Design review of the part built by this model. Coordinates are the model's own, in mm. Face numbers are marked on the shaded views. A direction names the side the tool comes from. Coordinates: 2 decimals unless noted, no trailing zeros. Write each loop counter-clockwise with the first axis right and the second up, starting at its lowest first coordinate (ties: lowest second). Pieces come first, ordered by that corner, then holes. Notation, with made-up numbers: (62, 26) - (75, 26) arc R28 cw to (75, 62) - close; hole circle Ø10 at (22, 3.5). An arc over 180 degrees is marked (long way). Answer as a JSON object with one key per item and string values.
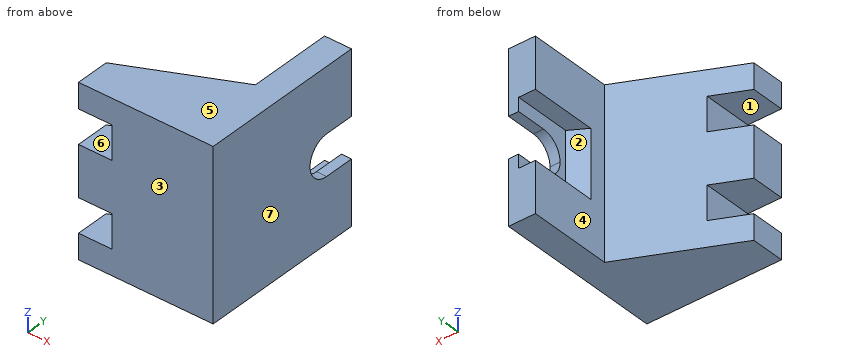
```python
from build123d import *

# Parameters (mm, degrees)
EXTRUDE_1_DEPTH          = 50
SKETCH_2_W               = 10
SKETCH_2_H               = 10
CUT_EXTRUDE_1_DEPTH      = 74.484692283
CUT_EXTRUDE_2_DEPTH      = 50
CUT_EXTRUDE_3_DEPTH      = 10
CUT_EXTRUDE_3_DEPTH_BACK = 10


with BuildPart() as part:
    # Эскиз1 → Бобышка-Вытянуть1 (new body)
    with BuildSketch(Plane.XY):
        Polygon((20, 25), (12, 25), (12, 0), (-20, -15), (-20, -25), (20, -25), align=None)
    extrude(amount=EXTRUDE_1_DEPTH)

    # Эскиз2 → Вырез-Вытянуть1 (cut, through all)
    with BuildSketch(Plane.XZ.offset(25)):
        with Locations((-15, 12.5)):
            Rectangle(SKETCH_2_W, SKETCH_2_H)
        with Locations((-15, 37.5)):
            Rectangle(SKETCH_2_W, SKETCH_2_H)
    extrude(amount=-CUT_EXTRUDE_1_DEPTH, mode=Mode.SUBTRACT)

    # Эскиз3 → Вырез-Вытянуть2 (cut)
    with BuildSketch(Plane(origin=(20, 0, 0), x_dir=(0, 0, -1), z_dir=(1, 0, 0))):
        with BuildLine():
            Line((-19, 25), (-25, 25))
            Line((-25, 25), (-25, 22))
            ThreePointArc((-25, 22), (-20.757359313, 20.242640687), (-19, 16))
            Line((-19, 16), (-19, 25))
        make_face()
        with BuildLine():
            ThreePointArc((-19, 16), (-20.757359313, 20.242640687), (-25, 22))
            Line((-25, 22), (-25, 10))
            ThreePointArc((-25, 10), (-20.757359313, 11.757359313), (-19, 16))
        make_face()
        with BuildLine():
            Line((-25, 10), (-25, 22))
            ThreePointArc((-25, 22), (-29.242640687, 20.242640687), (-31, 16))
            ThreePointArc((-31, 16), (-29.242640687, 11.757359313), (-25, 10))
        make_face()
        with BuildLine():
            Line((-25, 22), (-25, 25))
            Line((-25, 25), (-31, 25))
            Line((-31, 25), (-31, 16))
            ThreePointArc((-31, 16), (-29.242640687, 20.242640687), (-25, 22))
        make_face()
    extrude(amount=-CUT_EXTRUDE_2_DEPTH, mode=Mode.SUBTRACT)

    # Эскиз4 → Вырез-Вытянуть3 (cut, two sides: drawn at the far end of the back side and taken through both)
    with BuildSketch(Plane.XY.offset(25).offset(-CUT_EXTRUDE_3_DEPTH_BACK)):
        Polygon((12, 25), (12, 5), (17, 8), (17, 25), align=None)
    extrude(amount=CUT_EXTRUDE_3_DEPTH + CUT_EXTRUDE_3_DEPTH_BACK, mode=Mode.SUBTRACT)


solid = part.part
```
(1) The part is to be moulded in two halves that separate along Z. For the marked faces 5, 6 and 7, say which applies: pulls with the +Z half, pulls with the -Z half, needs draft (parallel to the pull), parting line crosses it, or undercut.
Solved:
{"face 5": "pulls with the +Z half", "face 6": "undercut", "face 7": "needs draft"}
(2) Take a section at C-C, the plane y = 13.5. Write out the cut boundary in (x, z).
Solved:
{"outline": "(12, 0) - (20, 0) - (20, 19.55) - (17, 19.55) - (17, 15) - (12, 15) - close; (12, 35) - (17, 35) - (17, 30.45) - (20, 30.45) - (20, 50) - (12, 50) - close"}
(3) Take a section at A-A, the plane y = -13.5. Write out the cut boundary in (x, z).
Solved:
{"outline": "(-16.8, 0) - (20, 0) - (20, 50) - (-16.8, 50) - (-16.8, 42.5) - (-10, 42.5) - (-10, 32.5) - (-16.8, 32.5) - (-16.8, 17.5) - (-10, 17.5) - (-10, 7.5) - (-16.8, 7.5) - close"}
(4) To check wall thickness, follow line 1 (Z direction, x = -12, y = -12); line 2 (Z direction, x = 15, y = 15.5); line 3 (Z direction, x = 18.5, y = 16). State the ranges of each line that lie inside material, in increasing order. Write a range as from..to.
Solved:
{"line 1": "z = 0..7.5, 17.5..32.5, 42.5..50", "line 2": "z = 0..15, 35..50", "line 3": "z = 0..19, 31..50"}
(5) Tool access review of the marked faces 1, 2, 3 and 4: name each direction out of +Z, -Z, +X, -X, +Y, -Y from which nothing blocks a thin tool from reaching the whole face with its end or side.
Solved:
{"face 1": "-X, +Y, -Y", "face 2": "-X, +Y", "face 3": "+Z, -Z, +X, -X, -Y", "face 4": "+Z, -Z, -X, +Y"}
(6) Take a section at D-D, the plane z = 40.5. Write out the cut boundary in (x, y), and give its area (3 significant figures).
Solved:
{"outline": "(-10, -25) - (20, -25) - (20, 25) - (12, 25) - (12, 0) - (-10, -10.31) - close", "area": "837 mm^2"}
(7) Take a section at B-B, the plane z = 16. Write out the cut boundary in (x, y), and give its area (3 significant figures).
Solved:
{"outline": "(-10, -25) - (20, -25) - (20, 25) - (17, 25) - (17, 8) - (12, 5) - (12, 0) - (-10, -10.31) - close", "area": "744 mm^2"}
(8) For pin 1 (4 mm diameter, centred on x = 7.5, z = 29.5, fed in from +Y); pin 2 (12.5 mm diameter, centred on y = 15.5, z = 19.5, fed in from -X); pin 3 (3 mm diameter, centred on y = -7, z = 26, fed in from -X), all flat-tipped, find the tip position at first contact; note any pin that passes through.
Solved:
{"pin 1": "stops at y = -1.17", "pin 2": "stops at x = 12", "pin 3": "stops at x = -6.13"}
